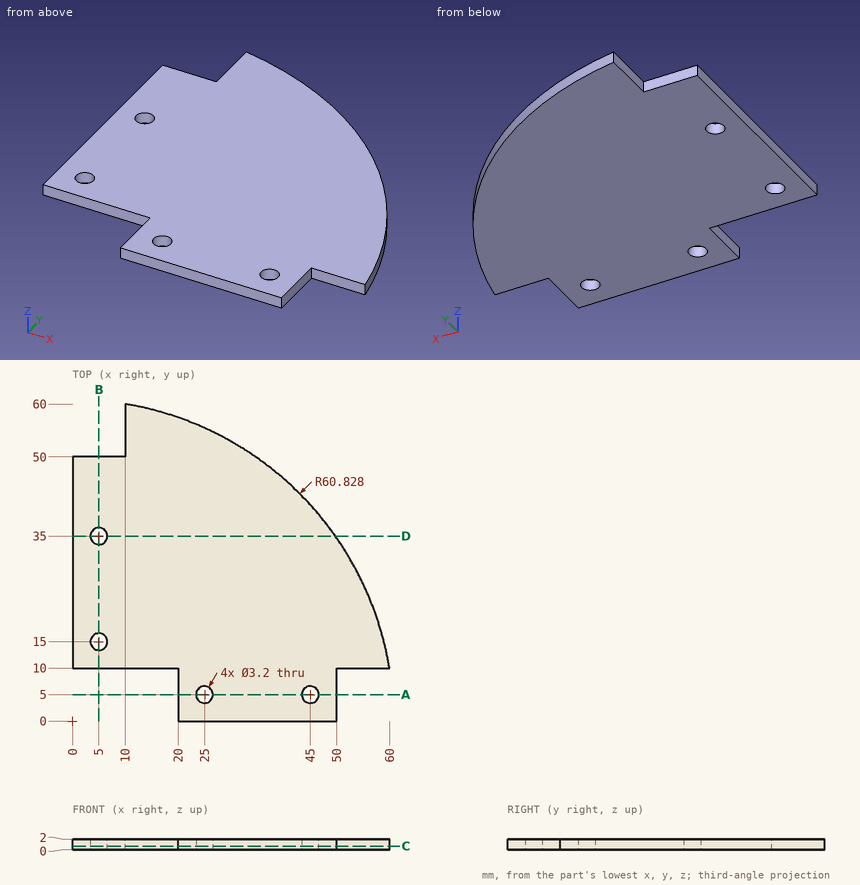
Drawing for the job (mm, zero at the part's lowest x, y, z). Coordinates: 2 decimals unless noted, no trailing zeros. Order: outer loops, then holes, each group sorted by start corner. A loop starts at its lowest first (then second) coordinate and runs counter-clockwise, first axis right, second up.
Item 1: Pin check, flat tip, straight feed: pin 1 Ø1 at (x, z) = (55, 1.5) entering from -Y. Stop position of the tip, or through.
Check sheet entries:
pin 1: stops at y = 10
Item 2: Band-saw the part on B-B on x = 5. List the corners of the cut face in (y, z).
Check sheet entries:
outline: (10, 0) - (13.4, 0) - (13.4, 2) - (10, 2) - close; (16.6, 0) - (33.4, 0) - (33.4, 2) - (16.6, 2) - close; (36.6, 0) - (50, 0) - (50, 2) - (36.6, 2) - close
Item 3: Band-saw the part on D-D on y = 35. List the corners of the cut face in (x, z).
Check sheet entries:
outline: (0, 0) - (3.4, 0) - (3.4, 2) - (0, 2) - close; (6.6, 0) - (49.75, 0) - (49.75, 2) - (6.6, 2) - close
Item 4: Band-saw the part on C-C on z = 0.65. List the corners of the cut face in (x, y) (1 decimal).
Check sheet entries:
outline: (0, 10) - (20, 10) - (20, 0) - (50, 0) - (50, 10) - (60, 10) arc R60.8 ccw to (10, 60) - (10, 50) - (0, 50) - close; hole circle Ø3.2 at (5, 15); hole circle Ø3.2 at (5, 35); hole circle Ø3.2 at (25, 5); hole circle Ø3.2 at (45, 5)
Item 5: Band-saw the part on A-A on y = 5. List the corners of the cut face in (x, z), plus the area to 3 significant figures.
Check sheet entries:
outline: (20, 0) - (23.4, 0) - (23.4, 2) - (20, 2) - close; (26.6, 0) - (43.4, 0) - (43.4, 2) - (26.6, 2) - close; (46.6, 0) - (50, 0) - (50, 2) - (46.6, 2) - close
area: 47.2 mm2
Item 6: Drill centre lines: L1, parallel to Y at x = 4, z = 1.4; L2, parallel to Y at x = 45, z = 0.65 (1 decimal); L3, parallel to Y at x = 8, z = 1.15. Where is each one in solid material? Low to high.
Check sheet entries:
L1: y = 10 to 13.75, 16.25 to 33.75, 36.25 to 50
L2: y = 0 to 3.4, 6.6 to 40.9
L3: y = 10 to 50
